```python
from build123d import *

# Parameters (mm, degrees)
SKETCH_1_R               = 10
EXTRUDE_1_DEPTH          = 5
SKETCH_2_R               = 7.952304339
EXTRUDE_2_DEPTH          = 10
EXTRUDE_2_TAPER          = 5
EXTRUDE_3_DEPTH          = 8
EXTRUDE_3_DEPTH_BACK     = 8
CUT_EXTRUDE_3_DEPTH      = 34.173609497
CUT_EXTRUDE_4_DEPTH      = 36.648067297
CUT_EXTRUDE_4_DEPTH_BACK = 36.648067297
SKETCH_12_R              = 8.616944053
EXTRUDE_4_DEPTH          = 1
SKETCH_13_W              = 5
SKETCH_13_H              = 1
CUT_EXTRUDE_5_DEPTH      = 5


with BuildPart() as part:
    # 草图1 → 拉伸1 (new body)
    with BuildSketch(Plane.XY):
        Circle(SKETCH_1_R)
    extrude(amount=EXTRUDE_1_DEPTH)

    # 草图2 → 拉伸2 (add)
    with BuildSketch(Plane.XY.offset(5)):
        Circle(SKETCH_2_R)
    extrude(amount=EXTRUDE_2_DEPTH, taper=EXTRUDE_2_TAPER)

    # 草图6 → 拉伸3 (add, two sides: drawn at the far end of the back side and taken through both)
    with BuildSketch(Plane(origin=(0, 0, 0), x_dir=(1, 0, 0), z_dir=(0, 1, 0)).offset(-EXTRUDE_3_DEPTH_BACK)):
        Polygon((0, -14.907325308), (-8.038553131, -14.907325308), (-8.038553131, -18), (11.857379423, -18), (27.26622564, -20.43963433), (27.897312043, -16.453662654), (12.347032914, -14.907325308), align=None)
    extrude(amount=EXTRUDE_3_DEPTH + EXTRUDE_3_DEPTH_BACK)

    # 草图10 → 切除-拉伸3 (cut, through all)
    with BuildSketch(Plane(origin=(0, 0, 14.907325308), x_dir=(-1, 0, 0), z_dir=(0, 0, -1))):
        with BuildLine():
            Line((8.038553131, 8), (0.481598082, 8))
            ThreePointArc((0.481598082, 8), (8.014482935, 0), (0.481598082, -8))
            Line((0.481598082, -8), (8.038553131, -8))
            Line((8.038553131, -8), (8.038553131, 8))
        make_face()
    extrude(amount=-CUT_EXTRUDE_3_DEPTH, mode=Mode.SUBTRACT)

    # 草图11 → 切除-拉伸4 (cut, two sides: drawn at the far end of the back side and taken through both)
    with BuildSketch(Plane(origin=(-2.490226462, 0, 15.728388526), x_dir=(0.9876971253210124, 0, 0.15637899038108757), z_dir=(-0.15637899038108757, 0, 0.9876971253210124)).offset(-CUT_EXTRUDE_4_DEPTH_BACK)):
        with BuildLine():
            Line((30.127102063, 8), (22.32671173, 8))
            ThreePointArc((22.32671173, 8), (27.854238113, 5.586727337), (30.127102063, 0))
            Line((30.127102063, 0), (30.127102063, 8))
        make_face()
        with BuildLine():
            Line((30.127102063, -8), (30.127102063, 0))
            ThreePointArc((30.127102063, 0), (27.854238113, -5.586727337), (22.32671173, -8))
            Line((22.32671173, -8), (30.127102063, -8))
        make_face()
    extrude(amount=CUT_EXTRUDE_4_DEPTH + CUT_EXTRUDE_4_DEPTH_BACK, mode=Mode.SUBTRACT)

    # 草图12 → 拉伸4 (add)
    with BuildSketch(Plane(origin=(0, 0, 0), x_dir=(-1, 0, 0), z_dir=(0, 0, -1))):
        with Locations(Location((0, 0, 0), (0, 0, 180))):
            Circle(SKETCH_12_R)
    extrude(amount=EXTRUDE_4_DEPTH)

    # 草图13 → 切除-拉伸5 (cut)
    with BuildSketch(Plane(origin=(0, 0, -1), x_dir=(-1, 0, 0), z_dir=(0, 0, -1))):
        Rectangle(SKETCH_13_W, SKETCH_13_H)
    extrude(amount=-CUT_EXTRUDE_5_DEPTH, mode=Mode.SUBTRACT)


solid = part.part
```
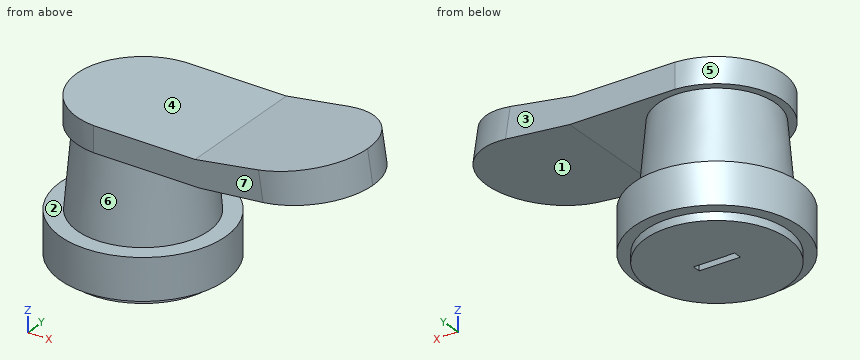
Geometry: final body of the model. Coordinates: model frame, mm. Face numbers are marked on the shaded views. A direction names the side the tool comes from. Coordinates: 2 decimals unless noted, no trailing zeros. Order: outer loops, then holes, each group sorted by start corner. A loop starts at its lowest first (then second) coordinate and runs counter-clockwise, first axis right, second up. Notation, with made-up numbers: (32, 8.5) -> (82, 8.5) arc R22 ccw to (82, 15.5) -> close; hole circle Ø10 at (-20.5, 37). An arc over 180 degrees is marked (long way). Answer in a Markdown table with one row per item.
Item 1: Section B-B on z = 10. Output: boundary loops of the cut face in (x, y), plus the area to 3 significant figures.
Return value:
| item | result |
|---|---|
| outline | circle Ø15.03 at (0, 0) |
| area | 177 mm² |
Item 2: Section C-C on x = 11. Output: boundary loops of the cut face in (y, z).
Return value:
| item | result |
|---|---|
| outline | (-8, 14.91) -> (8, 14.91) -> (8, 18) -> (-8, 18) -> close |
Item 3: Draft query along Z for the marked faces 1, 2 and 3. Return one class per face: released by +Z, released by -Z, zero draft, split by the parting line, or undercut.
Return value:
| item | result |
|---|---|
| face 1 | released by -Z |
| face 2 | undercut |
| face 3 | zero draft |
Item 4: Contact query for flat-ended pins moving along their axis: P1, Ø1.3, axis at x = 12.5, z = 16.5, coming from the -Y side; P2, Ø4.5, axis at x = 8, z = 17, coming from the +Y side; P3, Ø1, axis at x = 21, y = 1.5, coming from the +Z side. Output: stop coordinate, or through.
Return value:
| item | result |
|---|---|
| P1 | stops at y = -8 |
| P2 | stops at y = 8 |
| P3 | stops at z = 19.53 |
Item 5: Ray query, L1, parallel to Z at x = 2, y = -1; L2, parallel to Y at x = 1.5, z = 1.5; L3, parallel to Z at x = 5, y = -8.25. Return the intervals inside material, ascending.
Return value:
| item | result |
|---|---|
| L1 | z = -1 to 18 |
| L2 | y = -9.89 to -0.5, 0.5 to 9.89 |
| L3 | z = 0 to 5 |
Item 6: Section A-A on x = 0. Output: boundary loops of the cut face in (y, z).
Return value:
| item | result |
|---|---|
| outline | (-10, 0) -> (-8.62, 0) -> (-8.62, -1) -> (-0.5, -1) -> (-0.5, 4) -> (0.5, 4) -> (0.5, -1) -> (8.62, -1) -> (8.62, 0) -> (10, 0) -> (10, 5) -> (7.95, 5) -> (7.09, 14.91) -> (8, 14.91) -> (8, 18) -> (-8, 18) -> (-8, 14.91) -> (-7.09, 14.91) -> (-7.95, 5) -> (-10, 5) -> close |
Item 7: Section D-D on z = 6.5. Output: boundary loops of the cut face in (x, y).
Return value:
| item | result |
|---|---|
| outline | circle Ø15.64 at (0, 0) |
Item 8: Access query for the marked faces 4, 5, 6 and 7. Directions: +Z, -Z, +X, -X, +Y, -Y. A direction counts if a zero-diameter tool reaches every point of the face in a straight line with its end or side. Return the directions, or none.
Return value:
| item | result |
|---|---|
| face 4 | +Z, -X, +Y, -Y |
| face 5 | +Z, -X |
| face 6 | none |
| face 7 | +Z, +X, -X, -Y |
